from build123d import *

# Parameters (mm, degrees)
SKETCH_R  = 2.1
PAD_DEPTH = 3


with BuildPart() as part:
    # Sketch → Pad (new body)
    with BuildSketch(Plane.YZ):
        with BuildLine():
            ThreePointArc((-17.5, 19), (-21.035534, 17.535534), (-22.5, 14))
            ThreePointArc((-22.5, 14), (-21.531129, 11.04196), (-19, 9.230304))
            Line((-19, 9.230304), (-19, -1.5))
            Line((-19, -1.5), (22.5, -1.5))
            Line((22.5, 14), (22.5, -1.5))
            ThreePointArc((22.5, 14), (21.035534, 17.535534), (17.5, 19))
            Line((11, 19), (17.5, 19))
            ThreePointArc((11, 19), (7.464466, 17.535534), (6, 14))
            Line((6, 6), (6, 14))
            ThreePointArc((-6, 6), (0, 0), (6, 6))
            Line((-6, 6), (-6, 14))
            ThreePointArc((-6, 14), (-7.464466, 17.535534), (-11, 19))
            Line((-17.5, 19), (-11, 19))
        make_face()
        with Locations((-17.5, 14)):
            Circle(SKETCH_R, mode=Mode.SUBTRACT)
        with Locations((17.5, 14)):
            Circle(SKETCH_R, mode=Mode.SUBTRACT)
    extrude(amount=PAD_DEPTH)


solid = part.part
Can you work these out from the model? Positions are in its coordinate system, mm. A direction names the side the tool comes from. Coordinates: 2 decimals unless noted, no trailing zeros. Write each loop counter-clockwise with the first axis right and the second up, starting at its lowest first coordinate (ties: lowest second). Pieces come first, ordered by that corner, then holes.
Q1. If we mould it in two halves opening along Z, with no side actions, what happens to faces 4 (the face through (1.479, 19.503, 14.631)), 5 (the face through (1.479, -15.497, 14.631)), 6 (the face through (0, 5, 2)), 7 (the face through (1, 1, -1.5))? For each: +Z half, -Z half, draft (parallel to the pull), parting line (faces both ways), or undercut.
Results found:
face 4: undercut
face 5: undercut
face 6: draft
face 7: -Z half
Q2. Imagine slicing it at B-B, the plane z = 1.25. List the corners of the cut face in (x, y) for me, plus the area to 3 significant figures.
Results found:
outline: (0, -19) - (3, -19) - (3, -3.67) - (0, -3.67) - close; (0, 3.67) - (3, 3.67) - (3, 22.5) - (0, 22.5) - close
area: 103 mm2
Q3. Imagine slicing it at A-A, the plane x = 0.45. List the corners of the cut face in (y, z) for me, plus the area to 3 significant figures.
Results found:
outline: (-19, -1.5) - (22.5, -1.5) - (22.5, 14) arc R5 ccw to (17.5, 19) - (11, 19) arc R5 ccw to (6, 14) - (6, 6) arc R6 cw to (-6, 6) - (-6, 14) arc R5 ccw to (-11, 19) - (-17.5, 19) arc R5 ccw to (-19, 9.23) - close; hole circle Ø4.2 at (-17.5, 14); hole circle Ø4.2 at (17.5, 14)
area: 619 mm2
Q4. Please list where these lines run through material, in increasing order: L1, parallel to Z at x = 1.5, y = -17.5; L2, parallel to Y at x = 1.45, z = 12.75; L3, parallel to Y at x = 0.45, z = 8.75.
Results found:
L1: z = -1.5 to 11.9, 16.1 to 19
L2: y = -22.34 to -19.19, -15.81 to -6, 6 to 15.81, 19.19 to 22.5
L3: y = -19 to -6, 6 to 22.5
Q5. Imagine slicing it at D-D, the plane z = 11.5. List the corners of the cut face in (x, y) for me, plus the area to 3 significant figures.
Results found:
outline: (0, -21.83) - (3, -21.83) - (3, -6) - (0, -6) - close; (0, 6) - (3, 6) - (3, 22.5) - (0, 22.5) - close
area: 97.0 mm2
Q6. Which directions (+Z, -Z, +X, -X, +Y, -Y) give clear straight access to the entire face, cutting with the end or side of a thin tool? Please do faces 1 (the face through (1, 8, 18)), 2 (the face through (1, -19, 4)), 3 (the face through (1, 22.5, 6)).
Results found:
face 1: +Z, +X, -X
face 2: -Z, +X, -X, -Y
face 3: +Z, -Z, +X, -X, +Y
Q7. Imagine slicing it at C-C, the plane y = 0. List the corners of the cut face in (x, z) for me, plus the area to 3 significant figures.
Results found:
outline: (0, -1.5) - (3, -1.5) - (3, 0) - (0, 0) - close
area: 4.50 mm2
Q8. For P1, Ø2.5, axis at y = 17.5, z = 14, coming from the -X side; P2, Ø0.9, axis at x = 1, z = 8, coming from the -Y side, each with a flat end and sliding along its axis, tell me the tip position at first contact or that it passes through.
Results found:
P1: passes through
P2: stops at y = -19
